Autodesk Inventor part; units mm, degrees
ref_plane "YZ Plane" through (0, 0, 0) normal (1, 0, 0) x (0, 1, 0)
ref_plane "XZ Plane" through (0, 0, 0) normal (0, 1, 0) x (-1, 0, 0)
ref_plane "XY Plane" through (0, 0, 0) normal (0, 0, 1) x (1, 0, 0)
sketch "Sketch1" plane through (0, 0, 0) normal (0, 1, 0) x (-1, 0, 0)
  line L0 (0, 0) -> (0, 76.2)
  line L1 (0, 76.2) -> (25.4, 76.2)
  line L2 (25.4, 76.2) -> (25.4, 25.4)
  line L3 (25.4, 25.4) -> (76.2, 25.4)
  line L4 (76.2, 25.4) -> (76.2, 0)
  line L5 (76.2, 0) -> (0, 0)
  line L6 (25.4, 25.4) -> (0, 0) construction
  circle A0 centre (12.7, 63.5) radius 3.3782
  circle A1 centre (12.7, 25.4) radius 3.3782
  circle A2 centre (25.4, 12.7) radius 3.3782
  circle A3 centre (63.5, 12.7) radius 3.3782
  dimension "d0" = 76.2
  dimension "d1" = 25.4
  dimension "d2" = 50.8
  dimension "d3" = 50.8
  dimension "d4" = 25.4
  dimension "d5" = 6.7564
  dimension "d6" = 6.7564
  dimension "d7" = 6.7564
  dimension "d8" = 6.7564
  dimension "d9" = 12.7
  dimension "d10" = 0
  dimension "d11" = 12.7
  dimension "d12" = 12.7
  dimension "d13" = 12.7
  dimension "d14" = 12.7
  dimension "d15" = 12.7
extrude "Extrusion1" add sketch "Sketch1" along normal blind 3.175
sketch "Sketch2" plane through (0, 0, 0) normal (0, -1, 0) x (1, 0, 0)
  line L0 (0, 76.2) -> (0, 0)
  line L1 (0, 0) -> (-76.2, 0)
  line L2 (0, 25.4) -> (15.621, 25.4)
  line L3 (15.621, 25.4) -> (15.621, -12.7)
  line L4 (15.621, -12.7) -> (-9.779, -12.7)
  line L5 (-9.779, -12.7) -> (-9.779, 0)
  dimension "d19" = 15.621
  dimension "d20" = 38.1
  dimension "d21" = 25.4
extrude "Extrusion2" add sketch "Sketch2" against normal blind 3.175
sketch "Sketch3" plane through (0, 0, 0) normal (0, -1, 0) x (1, 0, 0)
  circle A0 centre (-63.5, 12.7) radius 3.3782
  circle A1 centre (-25.4, 12.7) radius 3.3782
  circle A2 centre (-12.7, 25.4) radius 3.3782
  circle A3 centre (-12.7, 63.5) radius 3.3782
  line L0 (0, 76.2) -> (0, 25.4)
  line L1 (-25.4, 76.2) -> (0, 76.2)
  line L2 (-25.4, 25.4) -> (-25.4, 76.2)
  line L3 (-76.2, 25.4) -> (-25.4, 25.4)
  line L4 (-76.2, 0) -> (-76.2, 25.4)
  line L5 (-9.779, 0) -> (-76.2, 0)
  line L6 (-9.779, 0) -> (-9.779, -12.7)
  line L7 (-9.779, -12.7) -> (15.621, -12.7)
  line L8 (15.621, -12.7) -> (15.621, 25.4)
  line L9 (15.621, 25.4) -> (0, 25.4)
  point P0 (0, 0)
properties part number "Gusset Connector"
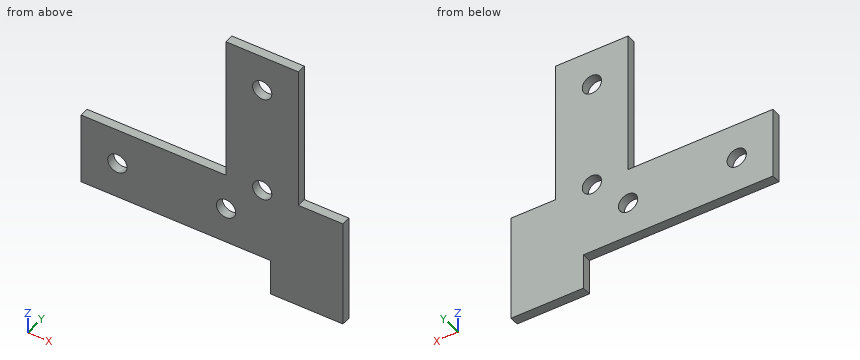
Could you check a few things on this model? Use its own coordinates, in mm. Round coordinates to 2 decimals unless told otherwise and drop trailing zeros. Write each loop counter-clockwise with the first axis right and the second up, starting at its lowest first coordinate (ties: lowest second). Pieces come first, ordered by that corner, then holes. Notation, with made-up numbers: (17.25, 62) - (40.25, 62) arc R13 cw to (40.25, 70) - close; hole circle Ø8 at (13.5, -23.5). An arc over 180 degrees is marked (long way). Put each result on its own line as item: value. Start each with the question number.
(1) I want a section at C-C, the plane y = 1.5. Please give me the cut outline in (x, z), plus the area to 3 significant figures.
(2) I want a section at B-B, the plane x = -63.5. Please give me the cut outline in (y, z) (3 decimals), plus the area to 3 significant figures.
(3) I want a section at A-A, the plane z = 12.7. Please give me the cut outline in (x, y) (3 decimals), plus the area to 3 significant figures.
(4) Will these pins go through, and if not, where does the flat tip stop? pin 1 (1 mm diameter, centred on x = -38, y = 2.5, fed in from -Z); pin 2 (1 mm diameter, centred on x = -45.5, y = 0.5, fed in from +Z).
(5) I want a section at D-D, the plane z = 63.5. Please give me the cut outline in (x, y) (3 decimals).
(6) I need wall thicknesses on probe 1 along Z at (x, y) = (-12.7, 1.5); probe 2 along Z at (x, y) = (-63.5, 1.45); probe 3 along X at (y, z) = (1.2, -1.5). Which ranges of each line are inside material? Lowest first, please.
Here are the results:
1. outline: (-76.2, 0) - (-9.78, 0) - (-9.78, -12.7) - (15.62, -12.7) - (15.62, 25.4) - (0, 25.4) - (0, 76.2) - (-25.4, 76.2) - (-25.4, 25.4) - (-76.2, 25.4) - close; hole circle Ø6.76 at (-63.5, 12.7); hole circle Ø6.76 at (-25.4, 12.7); hole circle Ø6.76 at (-12.7, 25.4); hole circle Ø6.76 at (-12.7, 63.5)
1. area: 3,800 mm^2
2. outline: (0, 0) - (3.175, 0) - (3.175, 9.322) - (0, 9.322) - close; (0, 16.078) - (3.175, 16.078) - (3.175, 25.4) - (0, 25.4) - close
2. area: 59.2 mm^2
3. outline: (-76.2, 0) - (-66.878, 0) - (-66.878, 3.175) - (-76.2, 3.175) - close; (-60.122, 0) - (-28.778, 0) - (-28.778, 3.175) - (-60.122, 3.175) - close; (-22.022, 0) - (15.621, 0) - (15.621, 3.175) - (-22.022, 3.175) - close
3. area: 249 mm^2
4. pin 1: stops at z = 0
4. pin 2: stops at z = 25.4
5. outline: (-25.4, 0) - (-16.078, 0) - (-16.078, 3.175) - (-25.4, 3.175) - close; (-9.322, 0) - (0, 0) - (0, 3.175) - (-9.322, 3.175) - close
6. probe 1: z = 0 to 22.02, 28.78 to 60.12, 66.88 to 76.2
6. probe 2: z = 0 to 9.32, 16.08 to 25.4
6. probe 3: x = -9.78 to 15.62
